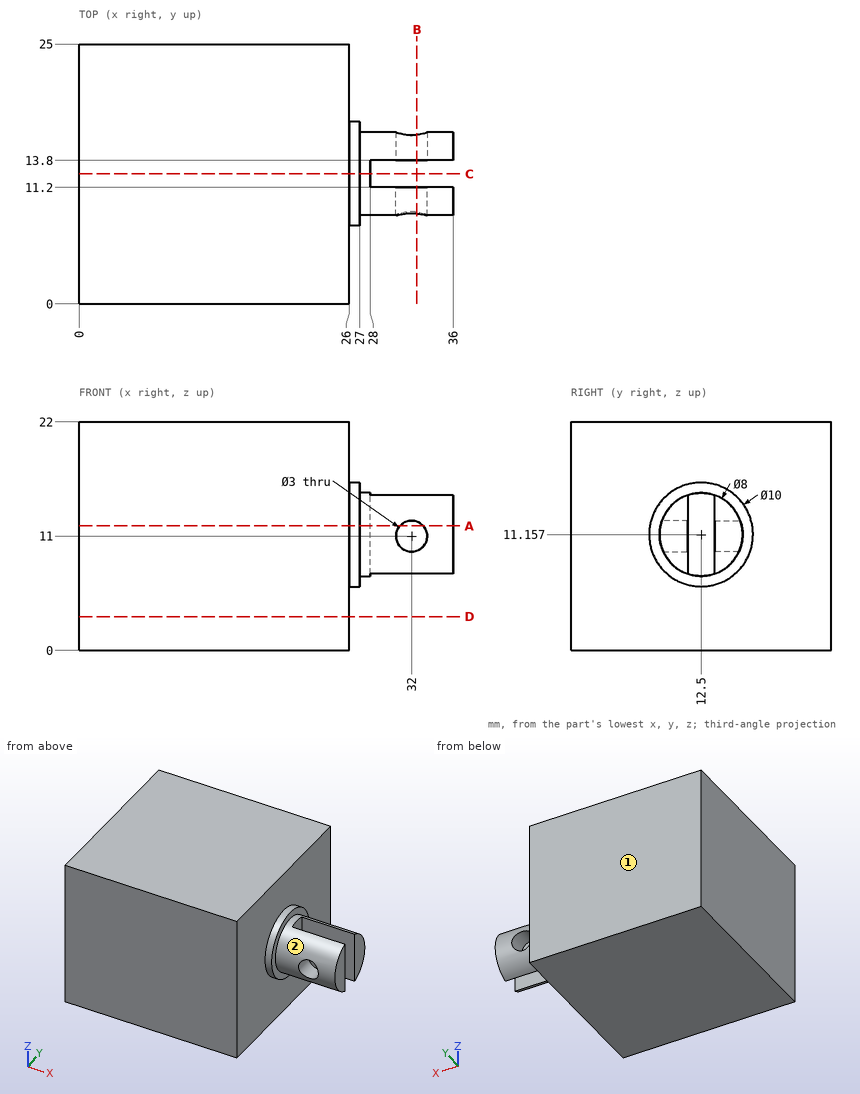
Geometry check sheet. Reference: drawing and pictorial views, mm from the part's lowest x, y, z. A direction names the side the tool comes from. Coordinates: 2 decimals unless noted, no trailing zeros. Loops run counter-clockwise (first coordinate to the right, second up) from the corner with the lowest first, then second, coordinate; pieces in that order, holes last. Notation, with made-up numbers: (33, 58.25) -> (40, 58.25) arc R19 ccw to (40, 64.25) -> close; hole circle Ø1 at (12, 74). An arc over 180 degrees is marked (long way). Write item = value, one per line. Start each with the question number.
1. Section check B-B on x = 32.5. Record the cut outline in (y, z) (1 decimal).
2. Section check C-C on y = 12.5. Record the cut outline in (x, z).
3. Depth check by flat-ended pin: P1, Ø8.5, axis at x = 33.5, z = 13, coming from the -Y side; P2, Ø3.5, axis at x = 32, z = 11, coming from the +Y side. Enter the tip coordinate at first touch or a pass-through.
4. Tool access check on the marked faces 1 and 2. Record the directions out of +Z, -Z, +X, -X, +Y, -Y that give a thin tool (end or side, any length) a straight path to the whole face; none if there is none.
5. Material ranges on line 1 (X direction, y = 10.1, z = 11); line 2 (X direction, y = 20.25, z = 18.5); line 3 (Z direction, x = 31, y = 15.5) (1 decimal), recorded low to high.
6. Section check A-A on z = 12. Record the cut outline in (x, y).
7. Section check D-D on z = 3.25. Record the cut outline in (x, y).
Responses:
q1.outline = (8.7, 12.4) -> (11.2, 12.4) -> (11.2, 14.9) arc R4 ccw to start; (8.8, 9.6) arc R4 ccw to (11.2, 7.4) -> (11.2, 9.6) -> close; (13.8, 7.4) arc R4 ccw to (16.2, 9.6) -> (13.8, 9.6) -> close; (13.8, 12.4) -> (16.3, 12.4) arc R4 ccw to (13.8, 14.9) -> close
q2.outline = (0, 0) -> (26, 0) -> (26, 6.16) -> (27, 6.16) -> (27, 7.16) -> (28, 7.16) -> (28, 15.16) -> (27, 15.16) -> (27, 16.16) -> (26, 16.16) -> (26, 22) -> (0, 22) -> close
q3.P1 = 8.5
q3.P2 = 16.5
q4.face_1 = +Z, -Z, +X, -X, +Y
q4.face_2 = +X
q5.line_1 = 0 to 30.5, 33.5 to 36
q5.line_2 = 0 to 26
q5.line_3 = 8.5 to 9.9, 12.1 to 13.8
q6.outline = (0, 0) -> (26, 0) -> (26, 7.57) -> (27, 7.57) -> (27, 8.59) -> (30.88, 8.59) -> (30.88, 11.2) -> (28, 11.2) -> (28, 13.8) -> (30.88, 13.8) -> (30.88, 16.41) -> (27, 16.41) -> (27, 17.43) -> (26, 17.43) -> (26, 25) -> (0, 25) -> close; (33.12, 8.59) -> (36, 8.59) -> (36, 11.2) -> (33.12, 11.2) -> close; (33.12, 13.8) -> (36, 13.8) -> (36, 16.41) -> (33.12, 16.41) -> close
q7.outline = (0, 0) -> (26, 0) -> (26, 25) -> (0, 25) -> close
